```python
from build123d import *

# Parameters (mm, degrees)
SKETCH2_R                   = 19.05
CUT_EXTRUDE1_DEPTH          = 185.94967748
SKETCH3_R                   = 28.575
SKETCH3_R_2                 = 25.4
CUT_EXTRUDE2_DEPTH          = 2.794
F_1_4_0_25_DIAMETER_HOLE1_D = 6.35


with BuildPart() as part:
    # Sketch1 → Revolve1 (revolve)
    with BuildSketch(Plane.XY, mode=Mode.PRIVATE) as revolve1_sk:
        with BuildLine():
            Line((0, 0), (0, 6.35))
            Line((0, 6.35), (-129.54, 6.35))
            Line((-129.54, 6.35), (-129.54, -19.05))
            Line((-129.54, -19.05), (-86.36, -19.05))
            Line((-86.36, -19.05), (-86.36, -16.51))
            ThreePointArc((-86.36, -16.51), (-81.524332957, -4.835667043), (-69.85, 0))
            Line((-69.85, 0), (0, 0))
        make_face()
    revolve(revolve1_sk.sketch.rotate(Axis((0, 0, 0), (0, 1, 0)), 270), axis=Axis((0, 0, 0), (0, 1, 0)))

    # Sketch2 → Cut-Extrude1 (cut, through all)
    with BuildSketch(Plane(origin=(0, 6.35, 0), x_dir=(1, 0, 0), z_dir=(0, 1, 0))):
        with Locations(Location((0, 0, 0), (0, 0, 270))):
            Circle(SKETCH2_R)
    extrude(amount=-CUT_EXTRUDE1_DEPTH, mode=Mode.SUBTRACT)

    # Sketch3 → Cut-Extrude2 (cut)
    with BuildSketch(Plane(origin=(0, 6.35, 0), x_dir=(1, 0, 0), z_dir=(0, 1, 0))):
        with Locations(Location((0, 0, 0), (0, 0, 270))):
            Circle(SKETCH3_R)
        with Locations(Location((0, 0, 0), (0, 0, 270))):
            Circle(SKETCH3_R_2, mode=Mode.SUBTRACT)
    extrude(amount=-CUT_EXTRUDE2_DEPTH, mode=Mode.SUBTRACT)

    # 1/4 (0.25) Diameter Hole1 (through all)
    with Locations(Plane(origin=(0, 6.35, -120.015), x_dir=(0, 0, 1), z_dir=(0, 1, 0))):
        with Locations((0, 0), (16.078961165, -60.0075), (60.0075, -103.936038835), (120.015, -120.015), (180.0225, -103.936038835), (223.951038835, -60.0075), (240.03, 0), (223.951038835, 60.0075), (180.0225, 103.936038835), (120.015, 120.015), (60.0075, 103.936038835), (16.078961165, 60.0075)):
            Hole(F_1_4_0_25_DIAMETER_HOLE1_D / 2)


solid = part.part
```
CAD build for the part. Positions are in the model's coordinates, mm. A direction names the side the tool comes from. Coordinates: 2 decimals unless noted, no trailing zeros. Order: outer loops, then holes, each group sorted by start corner. A loop starts at its lowest first (then second) coordinate and runs counter-clockwise, first axis right, second up.
(1) Pin check, flat tips, straight feed: pin 1 Ø8 at (y, z) = (-10, -84) entering from +X; pin 2 Ø3 at (x, y) = (-79.5, -1.5) entering from -Z; pin 3 Ø5 at (y, z) = (0, -75) entering from +X; pin 4 Ø10 at (x, z) = (0, 120.015) entering from -Y. Stop position of each tip, or through.
Solution:
pin 1: stops at x = 101.89
pin 2: stops at z = -103.42
pin 3: stops at x = 107.35
pin 4: stops at y = -19.05
(2) Drill centre lines: L1, parallel to Y at x = 37.5, z = 17; L2, parallel to Z at x = 23, y = -2; L3, parallel to Z at x = -2, y = -5. Where is each one in solid material? Low to high.
Solution:
L1: y = 0 to 6.35
L2: z = -127.48 to -74.25, 74.25 to 127.48
L3: z = -129.52 to -122.48, -117.55 to -81.66, 81.66 to 117.55, 122.48 to 129.52
(3) Which spindle directions (+Z, -Z, +X, -X, +Y, -Y) get a long thin tool onto all of the face, cutting with end or side? Do faces 4 (the face through (-107.036, -6.528, 60.696)), 5 (the face through (15, 0, -15)), 6 (the face through (-15.456, 4.973, -20.157)). Say none if no direction does.
Solution:
face 4: +Y, -Y
face 5: -Y
face 6: +Y
(4) Saw through at D-D, the plane z = -93. Write the cut outline in (x, y), and give its area (3 significant figures).
Solution:
outline: (-90.18, -19.05) - (90.18, -19.05) - (90.18, 6.35) - (-90.18, 6.35) - close
area: 4,580 mm2
(5) Mould opens along Z. For faces 1 (the face through (60.147, -6.528, 107.108)), 2 (the face through (0.954, -6.528, -123.043)), 3 (the face through (85, -19.05, -27)) say: released by +Z, released by -Z, zero draft, split by the parting line, or undercut.
Solution:
face 1: undercut
face 2: undercut
face 3: zero draft
(6) Saw through at A-A, the plane z = 0. Count the separate pieces of the cut face and the enclosed holes in it, and give its area (3 significant figures).
Solution:
separate pieces: 4
enclosed holes: 0
area: 2,830 mm2
